```python
from build123d import *

# Parameters (mm, degrees)
F2_T = -1.27


with BuildPart() as f1:
    # F0 (on Front) → F1 (revolve)
    with BuildSketch(Plane.XZ):
        Polygon((-3.175, -41.3657145261), (0, -41.3657145261), (0, 111.0342854739), (0, 130.0842854739), (-10.16, 130.0842854739), (-10.16, 114.2775136591), (-6.35, 110.4675136591), (-6.35, -36.8313446047), align=None)
    revolve(axis=Axis((0, 0, 34.8342854739), (0, 0, 1)))

    # F2
    f2_openings = [f1.faces().sort_by_distance(p)[0] for p in [
        (0, 0, 130.084285),
    ]]
    offset(amount=F2_T, openings=f2_openings, kind=Kind.INTERSECTION)


solid = f1.part
```
Design review of the part built by this model. Coordinates are the model's own, in mm. A direction names the side the tool comes from. Coordinates: 2 decimals unless noted, no trailing zeros. Loops run counter-clockwise (first coordinate to the right, second up) from the corner with the lowest first, then second, coordinate; pieces in that order, holes last. Notation, with made-up numbers: M 84.5,38 L 140.5,38 A33 cw 140.5,69 Z; hole C 69,28 d9. An arc over 180 degrees is marked long. One line per question, with ' | ' between items.
(1) Wall thickness on probe 1 along Y at (x, z) = (0, 118.25); probe 2 along Y at (x, z) = (0, 78.5): over which ranges is each line inside the solid? List them lowest first.
Filled in:
probe 1: y = -10.16 to -8.89, 8.89 to 10.16 | probe 2: y = -6.35 to -5.08, 5.08 to 6.35
(2) For pin 1 Ø10 at (x, z) = (-5.5, -20.5) entering from -Y; pin 2 Ø10 at (x, z) = (7.5, 22.5) entering from -Y; pin 3 Ø12 at (x, y) = (-2, 3.5) entering from +Z; pin 4 Ø1.5 at (x, y) = (3.5, 3) entering from +Z, all flat-tipped, find the tip position at first contact; note any pin that passes through.
Filled in:
pin 1: stops at y = -6.33 | pin 2: stops at y = -5.84 | pin 3: stops at z = 130.08 | pin 4: stops at z = 111.27
(3) We need section C-C (z = -5). Give the boundary of the cut face in (x, y), and give its area (3 significant figures).
Filled in:
outline: C 0,0 d12.7; hole C 0,0 d10.16 | area: 45.6 mm^2
(4) Machinability: for faces 1 (the face through (1.93, 8.68, 122.34)), 2 (the face through (1.38, 6.2, 35.79)), 3 (the face through (0, 0, -41.366)), which of the approach directions +Z, -Z, +X, -X, +Y, -Y give a long, thin tool a straight path to every point of the face, cutting with its end or side? Answer none if there is none.
Filled in:
face 1: +Z | face 2: -Z | face 3: -Z, +X, -X, +Y, -Y
(5) We need section A-A (y = 0). Give the boundary of the cut face in (x, z) (3 decimals), and give its area (3 significant figures).
Filled in:
outline: M -10.16,114.278 L -6.35,110.468 L -6.35,-36.831 L -3.175,-41.366 L 3.175,-41.366 L 6.35,-36.831 L 6.35,110.468 L 10.16,114.278 L 10.16,130.084 L 8.89,130.084 L 8.89,114.804 L 5.08,110.994 L 5.08,-36.431 L 2.514,-40.096 L -2.514,-40.096 L -5.08,-36.431 L -5.08,110.994 L -8.89,114.804 L -8.89,130.084 L -10.16,130.084 Z | area: 447 mm^2
